Autodesk Inventor part; units mm, degrees
ref_plane "YZ Plane" through (0, 0, 0) normal (1, 0, 0) x (0, 1, 0)
ref_plane "XZ Plane" through (0, 0, 0) normal (0, 1, 0) x (-1, 0, 0)
ref_plane "XY Plane" through (0, 0, 0) normal (0, 0, 1) x (1, 0, 0)
sketch "Sketch1" plane through (0, 0, 0) normal (0, 1, 0) x (-1, 0, 0)
  line L0 (0, -25.5) -> (-34.15, -25.5)
  line L1 (-34.15, -25.5) -> (-34.15, 0)
  line L2 (-34.15, 0) -> (-34.15, 25.5)
  line L3 (-34.15, 25.5) -> (0, 25.5)
  line L4 (0, 25.5) -> (34.15, 25.5)
  line L5 (34.15, 25.5) -> (34.15, 0)
  line L6 (34.15, 0) -> (34.15, -25.5)
  line L7 (34.15, -25.5) -> (0, -25.5)
  point P0 (0, 0)
extrude "Extrusion1" add sketch "Sketch1" along normal blind 7
sketch "Sketch3" plane through (-34.15, 0, 25.5) normal (0, 0, 1) x (1, 0, 0)
  line L0 (0, 0) -> (0, -78.85)
  point P0 (34.15, 0)
  dimension "d7" = 78.85
sketch "Sketch4" plane through (-34.15, 0, -25.5) normal (-1, 0, 0) x (0, 0, 1)
  line L0 (51, 0) -> (51, -78.85)
  line L1 (51, -78.85) -> (-39, -78.85)
  line L2 (-39, -78.85) -> (-39, -71.85)
  line L3 (0, 0) -> (-39, -71.85)
  line L4 (0, 0) -> (51, 0)
  point P0 (25.5, 0)
  dimension "d10" = 90
  dimension "d11" = 7
extrude "Extrusion2" add sketch "Sketch4" against normal blind 7
sketch "Sketch6" plane through (0, 7, 0) normal (0, 1, 0) x (1, 0, 0)
  line L0 (34.15, -25.5) -> (34.15, 25.5)
  line L1 (34.15, 25.5) -> (34.15, 0)
  line L2 (-34.15, 25.5) -> (-34.15, -25.5)
  circle A0 centre (8.15, 0) radius 5
  point P0 (0, 0)
  dimension "d20" = 10
extrude "Extrusion4" cut sketch "Sketch6" against normal blind 10
sketch "Sketch7" plane through (-27.15, 0, -25.5) normal (1, 0, 0) x (0, 0, -1)
  line L0 (-51, -78.85) -> (39, -78.85)
  line L1 (-51, -78.85) -> (39, -78.85)
  line L2 (39, -78.85) -> (39, -71.85)
  line L3 (39, -78.85) -> (39, -71.85)
  line L4 (39, -71.85) -> (-51, -71.85)
  line L5 (-51, 0) -> (-51, -78.85)
  line L6 (-51, -78.85) -> (-51, -71.85)
  point P0 (-25.5, 0)
sketch "Sketch8" plane through (0, 0, 0) normal (0, -1, 0) x (1, 0, 0)
  circle A0 centre (8.15, 0) radius 5
  line L0 (8.15, 18.5) -> (34.15, 18.5)
  line L1 (34.15, 25.5) -> (34.15, -25.5)
  line L2 (8.15, 25.5) -> (34.15, 25.5)
  line L3 (8.15, 25.5) -> (-27.15, 25.5)
  line L4 (-27.15, 25.5) -> (-27.15, -25.5)
  line L5 (8.15, 18.5) -> (-27.15, 18.5)
  line L6 (34.15, 25.5) -> (34.15, 18.5)
  line L7 (-27.15, 25.5) -> (-27.15, 18.5)
  point P0 (0, 0)
extrude "Extrusion6" add sketch "Sketch7" along normal blind 58.5
extrude "Extrusion7" add sketch "Sketch8" along normal blind 78.75 contours L5 L4 L3 L2 L1 L0
sketch "Sketch9" plane through (31.35, 0, -25.5) normal (1, 0, 0) x (0, 0, -1)
  line L0 (-51, -78.75) -> (-51, 7)
  line L1 (-44, 0) -> (-44, -71.85)
  line L2 (-51, -78.75) -> (-44, -78.75)
  line L3 (-44, -78.75) -> (-44, -71.85)
  line L4 (-44, -71.85) -> (-51, -71.85)
  line L5 (-51, -71.85) -> (-51, -78.75)
  point P0 (-25.5, 0)
extrude "Extrusion8" cut sketch "Sketch9" along normal blind 10
sketch "Sketch10" plane through (0, 7, 0) normal (0, 1, 0) x (1, 0, 0)
  point P0 (0, 0)
sketch "Boceto11" plane through (-34.15, -78.85, -64.5) normal (0, -1, 0) x (1, 0, 0)
  line L0 (72.0718, 89.9914) -> (72.0718, 37.9883)
  line L1 (72.0718, 37.9883) -> (65.5278, 37.9883)
  line L2 (65.5278, 37.9883) -> (65.5278, 89.9914)
  line L3 (72.0718, 89.9914) -> (72.0718, 92.1751)
  line L4 (72.0718, 92.1751) -> (65.5278, 92.1751)
  line L5 (65.5278, 92.1751) -> (65.5278, 89.9914)
  point P0 (34.15, 64.5)
extrude "Extrusión9" cut sketch "Boceto11" against normal blind 1000
sketch "Boceto18" plane through (-34.15, -78.85, 25.5) normal (0, 0, 1) x (1, 0, 0)
  point P0 (34.15, 78.85)
sketch "Boceto23" plane through (-27.15, 0, -25.5) normal (0, 0.4771, -0.8789) x (-1, 0, 0)
  point P0 (-27.15, 12.1648)
sketch "Boceto24" plane through (-27.15, 0, -25.5) normal (0, 0, -1) x (-1, 0, 0)
  line L0 (7, -71.85) -> (7, -78.85)
  line L1 (7, -78.35) -> (7, -78.85)
  line L2 (7, -78.85) -> (-58.5, -78.85)
  line L3 (-58.5, -78.85) -> (-58.5, -77.85)
  line L4 (-58.5, -71.85) -> (-58.5, -78.85)
  line L5 (-58.5, -77.85) -> (6, -77.85)
  line L6 (7, -77.85) -> (7, -78.85)
  line L7 (7, -78.85) -> (-58.8392, -78.85)
  line L8 (-58.5278, 7) -> (7, 7)
  line L9 (7, -78.85) -> (7, 7)
  line L10 (7, 7) -> (6, 7)
  line L11 (6, 6) -> (6, -77.85)
  line L12 (-58.5278, -71.85) -> (-58.5278, 7)
  line L13 (-58.5278, 7) -> (-58.5278, 6)
  line L14 (-58.5278, 6) -> (6, 6)
  line L15 (7, 0) -> (7, 7)
  line L16 (7, 6) -> (7, 7)
  line L17 (7, 7) -> (-58.5278, 7)
  point P0 (-27.15, 0)
  dimension "d65" = 1
  dimension "d66" = 1
  dimension "d67" = 1
extrude "Extrusión19" cut sketch "Boceto24" along normal mid plane 1000
sketch "Boceto25" plane through (31.35, -71.85, -64.5) normal (0, 0, -1) x (-1, 0, 0)
  point P0 (31.35, 71.85)
sketch "Boceto27" plane through (31.3778, 0, -25.5) normal (0, 0, -1) x (-1, 0, 0)
  line L0 (0, -71.85) -> (0, 6)
  line L1 (0, 6) -> (0.228, 6)
  line L2 (0, 6) -> (64.5278, 6)
  line L3 (0.228, 6) -> (0.228, -77.85)
  line L4 (0.0278, -77.85) -> (64.5278, -77.85)
  line L5 (0.0278, -71.85) -> (0.0278, -77.85)
  line L6 (0.228, -77.85) -> (0.0278, -77.85)
  line L7 (0.0278, -77.85) -> (0, 6)
  line L8 (0, 6) -> (0, -77.85)
  line L9 (0, -77.85) -> (0.0278, -77.85)
  point P0 (31.3778, 0)
  dimension "d73" = 0.228
extrude "Extrusión21" cut sketch "Boceto27" along normal mid plane 1000
sketch "Boceto28" plane through (-33.15, 0, -25.5) normal (-1, 0, 0) x (0, 0, 1)
  point P0 (25.5, 0)
sketch "Boceto30" plane through (-33.15, 0, -25.5) normal (-1, 0, 0) x (0, 0, 1)
  point P0 (25.5, 0)
sketch "Boceto31" plane through (-33.15, 0, -25.5) normal (-1, 0, 0) x (0, 0, 1)
  circle A0 centre (64.38, -38.5153) radius 2.6
  point P0 (25.5, 0)
  point P1 (64.38, -49.4573)
sketch "Boceto32" plane through (-27.15, -71.85, 18.5) normal (0, 1, 0) x (1, 0, 0)
  circle A0 centre (47, 71.5) radius 5
  circle A1 centre (47, 71.5) radius 5
  line L0 (52, 71.5) -> (58.2998, 71.5)
  line L1 (67, 83) -> (67, -7)
  line L2 (58.2998, -7) -> (-6, -7)
  line L3 (67, -7) -> (58.2998, -7)
  line L4 (58.2998, -7) -> (58.2998, 83)
  line L5 (47, 76.5) -> (47, 83)
  line L6 (-6, 83) -> (0, 83)
  line L7 (-6, 83) -> (-6, 91.5)
  line L8 (-6, 91.5) -> (67, 91.5)
  line L9 (67, 91.5) -> (67, 83)
  line L10 (-6, 83) -> (58.2998, 83)
  point P0 (27.15, 18.5)
extrude "Extrusión23" add sketch "Boceto32" against normal blind 6 contours L4 L10 L6 L7 L8 L9 L1 L3
sketch "Boceto33" plane through (-33.15, -77.85, 25.5) normal (-1, 0, 0) x (0, 0, 1)
  line L0 (0, 83.85) -> (0, 0)
  line L1 (0, 74.4354) -> (10.1255, 74.4354)
  line L2 (10.1255, 74.4354) -> (10.1255, 56.6115)
  line L3 (10.9445, 54.9975) -> (18.0243, 49.8171)
  line L4 (18.8039, 48.5979) -> (20.1084, 42.1205)
  line L5 (0, 11.6181) -> (18.1478, 11.6181)
  line L6 (20.1478, 13.6181) -> (20.1478, 41.7256)
  arc A0 (10.1255, 56.6115) -> (10.9445, 54.9975) centre (12.1255, 56.6115) ccw
  arc A1 (18.8039, 48.5979) -> (18.0243, 49.8171) centre (16.8433, 48.203) ccw
  arc A2 (20.1478, 41.7256) -> (20.1084, 42.1205) centre (18.1478, 41.7256) ccw
  arc A3 (18.1478, 11.6181) -> (20.1478, 13.6181) centre (18.1478, 13.6181) ccw
  point P0 (-25.5, 77.85)
  dimension "d91" = 2
extrude "Extrusión24" add sketch "Boceto33" against normal blind 6
extrude "Extrusión25" cut sketch "Boceto31" against normal blind 6
sketch "Boceto34" plane through (-27.15, -77.85, 25.5) normal (1, 0, 0) x (0, 0, -1)
  line L0 (-18.1478, 11.6181) -> (-21.8775, 11.6181)
  line L1 (-21.8775, 11.6181) -> (-21.8775, 48.067)
  line L2 (-21.8775, 48.067) -> (-10.1255, 56.8358)
  line L3 (-10.1255, 74.4354) -> (-10.1255, 56.6115)
  line L4 (-10.1255, 56.8358) -> (-10.1255, 48.9642)
  line L5 (-10.1255, 48.9642) -> (-16.6729, 42.1735)
  line L6 (-16.6729, 42.1735) -> (-18.1478, 11.6181)
  point P0 (25.5, 77.85)
extrude "Extrusión26" add sketch "Boceto34" against normal blind 6
fillet "Empalme5" radius 10 3 edges at (-30.15, -21.0142, 35.6255) (-30.15, -29.783, 47.3775) (-30.15, -66.2319, 47.3775)
sketch "Boceto37" plane through (-33.15, 6, 25.5) normal (0, 1, 0) x (1, 0, 0)
  circle A0 centre (41.3, 25.5) radius 6
  line L0 (41.3, 25.5) -> (17.3, 25.5)
  line L1 (17.3, 25.5) -> (17.3, 13.5)
  line L2 (17.3, 13.5) -> (17.3, 37.5)
  circle A1 centre (17.3, 13.5) radius 6
  circle A2 centre (17.3, 37.5) radius 6
  point P0 (33.15, 25.5)
  dimension "d106" = 24
  dimension "d107" = 12
  dimension "d108" = 24
  dimension "d109" = 12
  dimension "d110" = 12
extrude "Extrusión29" cut sketch "Boceto37" against normal blind 2.5 contours A1 | A2
sketch "Boceto39" plane through (-27.15, -71.85, 18.5) normal (0, 1, 0) x (1, 0, 0)
  line L0 (58.2998, -7) -> (58.2998, 0)
  line L1 (58.2998, 44) -> (58.2998, 91.5)
  line L2 (-6, 91.5) -> (67, 91.5)
  line L3 (0, 0) -> (58.2998, 0)
  line L4 (58.2998, 0) -> (58.2998, -7)
  line L5 (58.2998, -7) -> (67, -7)
  line L6 (58.2998, -7) -> (67, -7)
  line L7 (67, 91.5) -> (-6, 91.5)
  line L8 (67, -7) -> (67, 91.5)
  line L9 (67, 91.5) -> (58.2998, 91.5)
  line L10 (58.2998, 0) -> (58.2998, 44)
  point P0 (27.15, 18.5)
extrude "Extrusión31" cut sketch "Boceto39" against normal blind 10
sketch "Boceto41" plane through (-27.15, -71.85, 18.5) normal (0, 1, 0) x (1, 0, 0)
  line L0 (58.2998, 91.5) -> (58.2998, -7)
  line L1 (58.2998, 91.5) -> (31.7998, 91.5)
  line L2 (31.7998, 91.5) -> (31.7998, 65)
  line L3 (31.7998, 65) -> (58.2998, 65)
  line L4 (58.2998, 65) -> (58.2998, 91.5)
  circle A0 centre (31.7998, 65) radius 6
  point P0 (27.15, 18.5)
  dimension "d124" = 26.5
  dimension "d125" = 26.5
  dimension "d126" = 12
extrude "Extrusión32" cut sketch "Boceto41" against normal blind 10 contours A0 L2 L3 | L3 L2 A0
sketch "Sketch42" plane through (-27.15, -71.85, 18.5) normal (0, 1, 0) x (1, 0, 0)
  circle A0 centre (31.7998, 65) radius 6
  line L0 (31.7998, 71) -> (31.7998, 65)
  circle A1 centre (31.7998, 65) radius 18
  line L1 (0, 0) -> (0, 83)
  line L2 (0, 83) -> (31.7998, 83)
  line L3 (58.2998, 91.5) -> (-6, 91.5)
  line L4 (49.7998, 65) -> (49.7998, 0)
  line L5 (58.2998, 0) -> (0, 0)
  line L6 (0, 0) -> (58.2998, 0)
  line L7 (49.7998, 0) -> (58.2998, 0)
  line L8 (58.2998, 91.5) -> (58.2998, -7)
  line L9 (58.2998, 0) -> (58.2998, 91.5)
  line L10 (0, 83) -> (0, 44)
  line L11 (0, 83) -> (-6, 83)
  line L12 (-6, 91.5) -> (-6, 83)
  line L13 (-6, 83) -> (-6, 91.5)
  line L14 (58.2998, 91.5) -> (58.2998, 0)
  line L15 (-6, 91.5) -> (58.2998, 91.5)
  point P0 (27.15, 18.5)
  point P1 (58.2998, -7)
  dimension "d129" = 36
extrude "Extrusion33" cut sketch "Sketch42" against normal blind 10 contours A1 L2 L11 L12 L3 L8 L5 L4
sketch "Sketch43" plane through (-27.15, -71.85, 18.5) normal (0, 0, -1) x (-1, 0, 0)
  line L0 (6, -6) -> (-58.2998, -6)
  line L1 (0, 0) -> (-49.7998, 0)
  line L2 (-58.2998, -6) -> (-49.7998, -6)
  line L3 (-49.7998, -6) -> (-49.7998, 0)
  line L4 (-49.7998, 0) -> (-58.2998, 0)
  line L5 (-58.2998, 0) -> (-58.2998, -6)
  point P0 (-27.15, 71.85)
extrude "Extrusion34" add sketch "Sketch43" along normal blind 20
fillet "Fillet7" radius 7 1 edges at (31.1498, -74.85, -1.5)
fillet "Fillet8" radius 2 1 edges at (22.6498, -74.85, -1.5)
sketch "Sketch44" plane through (-33.15, 0, -25.5) normal (-1, 0, 0) x (0, 0, 1)
  line L0 (68.8577, -26.7837) -> (65.1452, -24.0136)
  line L1 (61.1255, -3.4146) -> (51, -3.4146)
  line L2 (65.1452, -24.0136) -> (51, -24.0136)
  line L3 (51, -24.0136) -> (51, -3.4146)
  line L4 (51, -3.4146) -> (65.1452, -3.4146)
  line L5 (65.1452, -3.4146) -> (65.1452, -24.0136)
  point P0 (25.5, 0)
extrude "Extrusion35" cut sketch "Sketch44" against normal blind 20
sketch "Sketch45" plane through (-33.15, 6, 25.5) normal (0, 1, 0) x (1, 0, 0)
  circle A0 centre (41.3, 25.5) radius 5
  circle A1 centre (41.3, 25.5) radius 4.25
  circle A2 centre (41.3, 25.5) radius 5
  point P0 (33.15, 25.5)
  dimension "d138" = 8.5
extrude "Extrusion36" add sketch "Sketch45" against normal blind 6
sketch "Sketch46" plane through (-33.15, 0, -25.5) normal (-1, 0, 0) x (0, 0, 1)
  line L0 (31, -77.85) -> (51, -77.85)
  line L1 (51, -77.85) -> (72.4185, -64.0875)
  line L2 (72.4185, -64.0875) -> (72.8775, -47.1091)
  line L3 (72.8775, -34.7985) -> (72.8775, -56.2319)
  line L4 (72.8775, -47.1091) -> (51, -38.5459)
  line L5 (51, -77.85) -> (51, 6)
  line L6 (51, -77.85) -> (51, -38.5459)
  line L7 (51, -77.85) -> (94.6859, -77.85)
  line L8 (94.6859, -77.85) -> (94.6859, -12.3032)
  line L9 (94.6859, -12.3032) -> (51, -12.3032)
  line L10 (51, -12.3032) -> (51, -77.85)
  point P0 (25.5, 0)
  point P1 (51, -12.3032)
extrude "Extrusion37" add sketch "Sketch46" along normal blind 9 and the other way blind 6 contours L5 L4 L2 L1
sketch "Sketch47" plane through (-42.15, -64.0875, 46.9185) normal (0, -0.027, 0.9996) x (1, 0, 0)
  point P0 (42.15, 62.7962)
sketch "Sketch48" plane through (-42.15, -64.0875, 46.9185) normal (0, -0.027, 0.9996) x (1, 0, 0)
  point P0 (42.15, 62.7962)
sketch "Sketch49" plane through (-42.15, -64.0875, 46.9185) normal (0, -0.027, 0.9996) x (1, 0, 0)
  line L0 (4.5153, 6.9733) -> (4.5153, 13.4811)
  line L1 (4.5153, 13.4811) -> (4.5153, 10.2272)
  line L2 (4.5153, 10.2272) -> (4.5153, 13.4811)
  line L3 (4.5153, 13.4811) -> (1.2539, 10.2272)
  line L4 (1.2539, 10.2272) -> (7.7617, 10.2272)
  circle A0 centre (4.5153, 10.2272) radius 3.2464
  point P0 (42.15, 62.7962)
extrude "Extrusion38" cut sketch "Sketch49" against normal blind 20 contours A0 L4 L0 | L0 L4 A0 | L4 A0 L3 L0 | L0 A0 L4 | A0 L3
extrude "Extrusion39" cut sketch "Sketch46" along normal mid plane 200 contours L1 L2 L4 L5 L9 L8 L7
properties part number "AC23[I3][R]" material "Aluminio 6061"
For this review, take the finished solid that the model builds, in its own axes (mm). A direction names the side the tool comes from. Round coordinates to 2 decimals unless told otherwise and drop trailing zeros. Order: outer loops, then holes, each group sorted by start corner. A loop starts at its lowest first (then second) coordinate and runs counter-clockwise, first axis right, second up. Notation, with made-up numbers: (69.5, -38) -> (117.5, -38) arc R15 ccw to (117.5, -16) -> close; hole circle Ø5 at (54, -0.75). An arc over 180 degrees is marked (long way). Use a Markdown table: item, result.
Item 1: Take a section at D-D (z = 0). State the section outline as (x, y) points, plus the area to 3 significant figures.
Resolved:
| item | result |
|---|---|
| outline | (-33.15, -77.85) -> (28.48, -77.85) -> (28.48, -71.85) -> (-27.15, -71.85) -> (-27.15, 0) -> (3.9, 0) -> (3.9, 6) -> (-33.15, 6) -> close; (12.4, 0) -> (31.15, 0) -> (31.15, 6) -> (12.4, 6) -> close |
| area | 1,140 mm² |
Item 2: For line 1 along Z through (x, y) = (-15.85, 4.75); line 2 along X through (y, z) = (3, 0); line 3 along Y through (x, z) = (-21.5, -3), list the stretches that pass through material, from the lowest coordinate up. Write a range as [from, to].
Resolved:
| item | result |
|---|---|
| line 1 | z = [-25.5, -18], [-6, 6], [18, 25.5] |
| line 2 | x = [-33.15, 3.9], [12.4, 31.15] |
| line 3 | y = [-77.85, -71.85], [0, 6] |
Item 3: Take a section at A-A (x = -15.85). State the section outline as (y, z) points, plus the area to 3 significant figures.
Resolved:
| item | result |
|---|---|
| outline | (-77.85, -64.5) -> (-71.85, -64.5) -> (-71.85, 18.5) -> (0, 18.5) -> (0, -25.5) -> (6, -25.5) -> (6, -18) -> (3.5, -18) -> (3.5, -6) -> (6, -6) -> (6, 6) -> (3.5, 6) -> (3.5, 18) -> (6, 18) -> (6, 25.5) -> (-77.85, 25.5) -> close |
| area | 1,290 mm² |
Item 4: Take a section at B-B (z = -12). State the section outline as (x, y) points.
Resolved:
| item | result |
|---|---|
| outline | (-33.15, -77.85) -> (22.65, -77.85) -> (22.65, -71.85) -> (-27.15, -71.85) -> (-27.15, 0) -> (31.15, 0) -> (31.15, 6) -> (-9.85, 6) -> (-9.85, 3.5) -> (-21.85, 3.5) -> (-21.85, 6) -> (-33.15, 6) -> close |
Item 5: Machinability: for faces 1 (the cylindrical face through (-17.151, 4.768, -6.143)), 2 (the flat face through (22.65, -75, -25)), 3 (the flat face through (2, 0, -4)), 4 (the flat face through (-1, 6, 0)), which of the approach directions +Z, -Z, +X, -X, +Y, -Y give a long, thin tool a straight path to every point of the face, cutting with its end or side? Answer none if there is none.
Resolved:
| item | result |
|---|---|
| face 1 | +Y |
| face 2 | -Z, +X, -Y |
| face 3 | -Z, +X |
| face 4 | +Z, -Z, +X, -X, +Y |
Item 6: Draft analysis for pull direction Z (two halves, no side actions). For faces 5 (the cylindrical face through (-0.11, -74.81, -42.85)), 6 (the cylindrical face through (-16.63, 4.77, 6.05)), 7 (the flat face through (-1, 3, -25.5)), 8 (the flat face through (-27.15, -58, 34)), state which applies: +Z half, -Z half, draft (parallel to the pull), parting line (faces both ways), or undercut.
Resolved:
| item | result |
|---|---|
| face 5 | undercut |
| face 6 | undercut |
| face 7 | -Z half |
| face 8 | draft |
Item 7: Take a section at C-C (x = 8.15). State the section outline as (y, z) points.
Resolved:
| item | result |
|---|---|
| outline | (-77.85, -64.16) -> (-71.85, -64.16) -> (-71.85, -51.37) -> (-77.85, -51.37) -> close; (-77.85, -41.63) -> (-71.85, -41.63) -> (-71.85, 18.5) -> (0, 18.5) -> (0, 4.25) -> (6, 4.25) -> (6, 25.5) -> (-77.85, 25.5) -> close; (0, -25.5) -> (6, -25.5) -> (6, -4.25) -> (0, -4.25) -> close |
Item 8: For pin 1 (7 mm diameter, centred on x = -37.5, y = -61, fed in from -Z); pin 2 (6 mm diameter, centred on y = -69, z = -27, fed in from +X); pin 3 (1 mm diameter, centred on x = -7, y = -15, fed in from +Z), all flat-tipped, find the tip position at first contact; note any pin that passes through.
Resolved:
| item | result |
|---|---|
| pin 1 | stops at z = 25.5 |
| pin 2 | stops at x = 22.65 |
| pin 3 | stops at z = 25.5 |
